The listing builds one solid part. Answer for the finished solid, in the listing's coordinates (mm). Face numbers are marked on the shaded views. A direction names the side the tool comes from. Give positions to 0.01 mm unless a question says otherwise; leave off trailing zeros. Write each loop counter-clockwise with the first axis right and the second up, starting at its lowest first coordinate (ties: lowest second). Pieces come first, ordered by that corner, then holes. Notation, with made-up numbers: (40.25, -20.5) - (77.25, -20.5) arc R17 cw to (77.25, 11.5) - close; hole circle Ø6 at (-39, 58). An arc over 180 degrees is marked (long way). Answer as CSV lines item,"result". Start each with the question number.
(1) For the marked faces 5 and 6, determine the directions among +Z, -Z, +X, -X, +Y, -Y from which every point of the face is accessible in a straight line to the end or side of a thin tool.
(2) Find section B-B (x = 11). Write down the section's boundary in (y, z).
(3) Find section A-A (y = 11.5). Write down the section's boundary in (x, z), then the cut area to 3 significant figures.
(4) Straight lines are drawn through the part: probe 1 along Y at (x, z) = (9.75, 0.8); probe 2 along Y at (x, z) = (8.25, 2.95); probe 3 along Y at (x, z) = (8.75, 1.05). For each, find the intervals that lie inside material, in ascending order.
(5) For a pull along X with two mould halves and no side action, classify the marked faces 1, 2, 3 and 4 as pulls with the +X half, pulls with the -X half, needs draft (parallel to the pull), parting line crosses it, or undercut.
(6) This flat-tipped pin is pushed along its axis until it touches: pin 1 Ø1.8 at (x, y) = (9.651, 3.682) entering from +Z. Where does it stop, or does it pass through?
(7) Find section C-C (z = 1.65). Write down the section's boundary in (x, y), then the cut area to 3 significant figures.
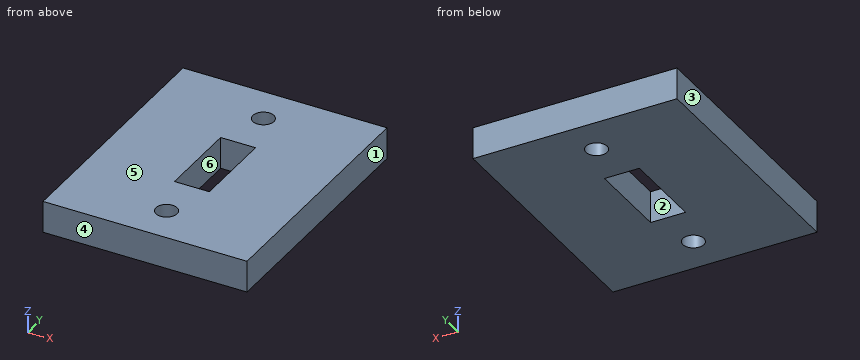
from build123d import *

# Parameters (mm, degrees)
SKETCH1_W           = 19.302
SKETCH1_H           = 23.874
SKETCH1_W_2         = 3.302
SKETCH1_H_2         = 7.874
BOSS_EXTRUDE1_DEPTH = 3
SKETCH3_R           = 1
CUT_EXTRUDE1_DEPTH  = 4


with BuildPart() as part:
    # Sketch1 → Boss-Extrude1 (new body)
    with BuildSketch(Plane.XY):
        with Locations((9.651, 11.937)):
            Rectangle(SKETCH1_W, SKETCH1_H)
        with Locations((9.651, 11.937)):
            Rectangle(SKETCH1_W_2, SKETCH1_H_2, mode=Mode.SUBTRACT)
    extrude(amount=BOSS_EXTRUDE1_DEPTH)

    # Sketch3 → Cut-Extrude1 (cut, through all)
    with BuildSketch(Plane(origin=(0, 0, 0), x_dir=(-1, 0, 0), z_dir=(0, 0, -1))):
        with Locations((-9.651, 20.192)):
            Circle(SKETCH3_R)
        with Locations((-9.651, 3.682)):
            Circle(SKETCH3_R)
    extrude(amount=-CUT_EXTRUDE1_DEPTH, mode=Mode.SUBTRACT)


solid = part.part
Result set:
1,face 5,"+Z, +X, -X, +Y, -Y"
1,face 6,"+Z, -Z"
2,outline,"(0, 0) - (8, 0) - (8, 3) - (0, 3) - close; (15.87, 0) - (23.87, 0) - (23.87, 3) - (15.87, 3) - close"
3,outline,"(0, 0) - (8, 0) - (8, 3) - (0, 3) - close; (11.3, 0) - (19.3, 0) - (19.3, 3) - (11.3, 3) - close"
3,area,"48.0 mm^2"
4,probe 1,"0 to 2.69, 4.68 to 8, 15.87 to 19.2, 21.19 to 23.87"
4,probe 2,"0 to 8, 15.87 to 23.87"
4,probe 3,"0 to 3.25, 4.12 to 8, 15.87 to 19.76, 20.63 to 23.87"
5,face 1,"pulls with the +X half"
5,face 2,"undercut"
5,face 3,"pulls with the -X half"
5,face 4,"needs draft"
6,pin 1,"through"
7,outline,"(0, 0) - (19.3, 0) - (19.3, 23.87) - (0, 23.87) - close; hole (8, 8) - (11.3, 8) - (11.3, 15.87) - (8, 15.87) - close; hole circle Ø2 at (9.65, 3.68); hole circle Ø2 at (9.65, 20.19)"
7,area,"429 mm^2"
